Could you check a few things on this model? Use its own coordinates, in mm. A direction names the side the tool comes from. Round coordinates to 2 decimals unless told otherwise and drop trailing zeros. Write each loop counter-clockwise with the first axis right and the second up, starting at its lowest first coordinate (ties: lowest second). Pieces come first, ordered by that corner, then holes. Notation, with made-up numbers: (68, -9) -> (101, -9) arc R17 ccw to (101, 23) -> close; hole circle Ø4 at (-24, 2.25). An arc over 180 degrees is marked (long way). Answer in a Markdown table with one row per item.
from build123d import *

# Parameters (mm, degrees)
SKETCH_W        = 100
SKETCH_H        = 45
PAD_DEPTH       = 45
SKETCH001_W     = 96
SKETCH001_H     = 41
POCKET_DEPTH    = 43
SKETCH002_W     = 10
SKETCH002_H     = 10
PAD001_DEPTH    = 9
SKETCH003_R     = 3
POCKET001_DEPTH = 3
SKETCH004_R     = 1.75
POCKET002_DEPTH = 42.001
SKETCH005_W     = 2
SKETCH005_H     = 20
POCKET003_DEPTH = 30
SKETCH006_W     = 10
SKETCH006_H     = 30
PAD002_DEPTH    = 13
SKETCH007_R     = 1.25
POCKET004_DEPTH = 12
SKETCH008_W     = 2
SKETCH008_H     = 7
POCKET005_DEPTH = 30


with BuildPart() as part:
    # Sketch → Pad (new body)
    with BuildSketch(Plane.XY):
        Rectangle(SKETCH_W, SKETCH_H)
    extrude(amount=PAD_DEPTH)

    # Sketch001 (on Face6 of Pad) → Pocket (cut)
    with BuildSketch(Plane.XY.offset(45)):
        Rectangle(SKETCH001_W, SKETCH001_H)
    extrude(amount=-POCKET_DEPTH, mode=Mode.SUBTRACT)

    # Sketch002 (on Face11 of Pocket) → Pad001 (join)
    with BuildSketch(Plane.XY.offset(2)):
        with Locations((15, -1.5)):
            Rectangle(SKETCH002_W, SKETCH002_H)
        with Locations((-15, 10)):
            Rectangle(SKETCH002_W, SKETCH002_H)
        with Locations((-15, -10)):
            Rectangle(SKETCH002_W, SKETCH002_H)
    extrude(amount=PAD001_DEPTH)

    # Sketch003 (on Face4 of Pad001) → Pocket001 (cut)
    with BuildSketch(Plane(origin=(0, 0, 0), x_dir=(1, 0, 0), z_dir=(0, 0, -1))):
        with Locations((15, 1.5)):
            Circle(SKETCH003_R)
    extrude(amount=-POCKET001_DEPTH, mode=Mode.SUBTRACT)

    # Sketch004 (on Face12 of Pocket001) → Pocket002 (cut, through all)
    with BuildSketch(Plane(origin=(0, 0, 3), x_dir=(1, 0, 0), z_dir=(0, 0, -1))):
        with Locations((15, 1.5)):
            Circle(SKETCH004_R)
    extrude(amount=-POCKET002_DEPTH, mode=Mode.SUBTRACT)

    # Sketch005 (on Face5 of Pocket002) → Pocket003 (cut)
    with BuildSketch(Plane.XY.offset(45)):
        with Locations((49, 0)):
            Rectangle(SKETCH005_W, SKETCH005_H)
    pocket003 = extrude(amount=-POCKET003_DEPTH, mode=Mode.SUBTRACT)

    # Mirrored: Pocket003 across YZ
    add(pocket003.mirror(Plane.YZ), mode=Mode.SUBTRACT)

    # Sketch006 (on Face20 of Mirrored) → Pad002 (join)
    with BuildSketch(Plane.XY.offset(2)):
        with Locations((43, 0)):
            Rectangle(SKETCH006_W, SKETCH006_H)
    extrude(amount=PAD002_DEPTH)

    # Sketch007 (on Face20 of Pad002) → Pocket004 (cut)
    with BuildSketch(Plane.XY.offset(15)):
        with Locations((40.5, 10)):
            Circle(SKETCH007_R)
        with Locations((40.5, -10)):
            Circle(SKETCH007_R)
    extrude(amount=-POCKET004_DEPTH, mode=Mode.SUBTRACT)

    # Sketch008 (on Face9 of Pocket004) → Pocket005 (cut)
    with BuildSketch(Plane.XY.offset(45)):
        with Locations((-49, 13.5)):
            Rectangle(SKETCH008_W, SKETCH008_H)
    extrude(amount=-POCKET005_DEPTH, mode=Mode.SUBTRACT)


solid = part.part
1) Imagine slicing it at A-A, the plane z = 8. Please give me the cut outline in (x, y).
Findings:
| item | result |
|---|---|
| outline | (-50, -22.5) -> (50, -22.5) -> (50, 22.5) -> (-50, 22.5) -> close; (-20, -15) -> (-10, -15) -> (-10, -5) -> (-20, -5) -> close; (-20, 5) -> (-10, 5) -> (-10, 15) -> (-20, 15) -> close; (10, -6.5) -> (20, -6.5) -> (20, 3.5) -> (10, 3.5) -> close; hole (-48, -20.5) -> (48, -20.5) -> (48, -15) -> (38, -15) -> (38, 15) -> (48, 15) -> (48, 20.5) -> (-48, 20.5) -> close; hole circle Ø3.5 at (15, -1.5); hole circle Ø2.5 at (40.5, -10); hole circle Ø2.5 at (40.5, 10) |
2) Imagine slicing it at B-B, the plane y = -1.5. Please give me the cut outline in (x, z).
Findings:
| item | result |
|---|---|
| outline | (-50, 0) -> (12, 0) -> (12, 3) -> (13.25, 3) -> (13.25, 11) -> (10, 11) -> (10, 2) -> (-48, 2) -> (-48, 15) -> (-50, 15) -> close; (16.75, 3) -> (18, 3) -> (18, 0) -> (50, 0) -> (50, 15) -> (38, 15) -> (38, 2) -> (20, 2) -> (20, 11) -> (16.75, 11) -> close |
3) For faces 5 (the face through (-1, -20.5, 24)), 6 (the face through (-1, 0, 0)), 7 (the face through (49, -10, 30)), 8 (the face through (-49, 17, 30)), which set-ups out of +Z, -Z, +X, -X, +Y, -Y let a thin tool reach every point of the face, with its end or its side?
Findings:
| item | result |
|---|---|
| face 5 | +Z |
| face 6 | -Z, +X, -X, +Y, -Y |
| face 7 | +Z, +X, -X |
| face 8 | +Z, -X |
4) Please list where these lines run through material, in increasing order: line 1 (Y direction, x = 15, z = 5); line 2 (Y direction, x = 15, z = 2.15); line 3 (X direction, y = -1.5, z = 2.2).
Findings:
| item | result |
|---|---|
| line 1 | y = -22.5 to -20.5, -6.5 to -3.25, 0.25 to 3.5, 20.5 to 22.5 |
| line 2 | y = -22.5 to -20.5, -6.5 to -4.5, 1.5 to 3.5, 20.5 to 22.5 |
| line 3 | x = -50 to -48, 10 to 12, 18 to 20, 38 to 50 |
5) For pin 1 (1.6 mm diameter, centred on x = -49, y = 1.5, fed in from +Z); pin 2 (3 mm diameter, centred on x = 17, y = -2, fed in from +Z); pin 3 (1 mm diameter, centred on x = -22, y = -5, fed in from +Z), each with a flat end and sliding along its axis, tell me the tip position at first contact or that it passes through.
Findings:
| item | result |
|---|---|
| pin 1 | stops at z = 15 |
| pin 2 | stops at z = 11 |
| pin 3 | stops at z = 2 |
6) Imagine slicing it at C-C, the plane z = 40.5. Please give me the cut outline in (x, y).
Findings:
| item | result |
|---|---|
| outline | (-50, -22.5) -> (50, -22.5) -> (50, -10) -> (48, -10) -> (48, -20.5) -> (-48, -20.5) -> (-48, -10) -> (-50, -10) -> close; (-50, 17) -> (-48, 17) -> (-48, 20.5) -> (48, 20.5) -> (48, 10) -> (50, 10) -> (50, 22.5) -> (-50, 22.5) -> close |
7) Imagine slicing it at D-D, the plane x = 15. Please give me the cut outline in (y, z).
Findings:
| item | result |
|---|---|
| outline | (-22.5, 0) -> (-4.5, 0) -> (-4.5, 3) -> (-3.25, 3) -> (-3.25, 11) -> (-6.5, 11) -> (-6.5, 2) -> (-20.5, 2) -> (-20.5, 45) -> (-22.5, 45) -> close; (0.25, 3) -> (1.5, 3) -> (1.5, 0) -> (22.5, 0) -> (22.5, 45) -> (20.5, 45) -> (20.5, 2) -> (3.5, 2) -> (3.5, 11) -> (0.25, 11) -> close |
8) Thinking about a two-plate mould opening in Y: for faces 1 (the face through (-1, 22.5, 22)), 2 (the face through (-8, -21, 45)), 3 (the face through (-15, 15, 6)), 4 (the face through (48, -15, 29)), which applies, +Y half, -Y half, draft (parallel to the pull), parting line (faces both ways), or undercut?
Findings:
| item | result |
|---|---|
| face 1 | +Y half |
| face 2 | draft |
| face 3 | undercut |
| face 4 | undercut |
